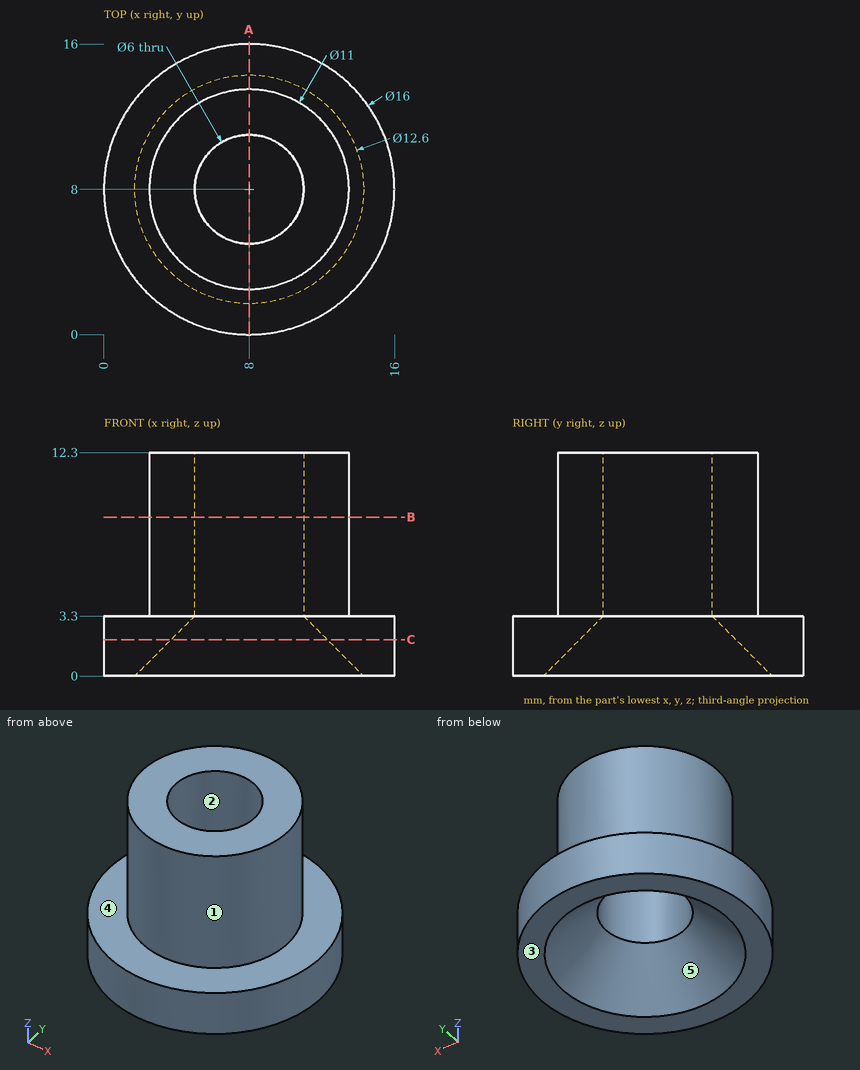
Print and shaded views of the part. All mm, measured from the part's lowest x, y and z. A direction names the side the tool comes from. Round coordinates to 2 decimals unless told otherwise and drop trailing zeros. Write each loop counter-clockwise with the first axis right and the second up, starting at its lowest first coordinate (ties: lowest second). Pieces come first, ordered by that corner, then holes.
(1) Probe line 1 along Y through (x, z) = (8, 7.25); line 2 along Z through (x, y) = (9.5, 15.25); line 3 along Y through (x, z) = (9.75, 4.75). List the from-to ranges inside material, lowest first.
(2) 3-axis set-ups, long thin cutter, end or side, ignore diameter. For the marked faces 4 and 5: which of +Z, -Z, +X, -X, +Y, -Y reach the whole face in a straight line?
(3) Mould opens along X. For the marked faces 1, 2 and 3 say: pulls with the +X half, pulls with the -X half, needs draft (parallel to the pull), parting line crosses it, or undercut.
(4) Slice it at C-C, the plane z = 2. Write the cut outline in (x, y).
(5) Slice it at A-A, the plane x = 8. Write the cut outline in (y, z).
(6) Drop flat-ended pins along their axis: P1, Ø3, axis at x = 10.5, z = 2, coming from the +Y side; P2, Ø2, axis at x = 2, z = 7, coming from the -Y side; P3, Ø2, axis at x = 8, y = 6.5, coming from the +Z side; P4, Ø2, axis at x = 8, z = 10.5, coming from the -Y side. Give the stop position or say it passes through.
(7) Slice it at B-B, the plane z = 8.75. Write the cut outline in (x, y).
From the geometry:
1. line 1: y = 2.5 to 5, 11 to 13.5
1. line 2: z = 0 to 3.3
1. line 3: y = 2.79 to 5.56, 10.44 to 13.21
2. face 4: +Z
2. face 5: -Z
3. face 1: parting line crosses it
3. face 2: undercut
3. face 3: needs draft
4. outline: circle Ø16 at (8, 8); hole circle Ø8.6 at (8, 8)
5. outline: (0, 0) - (1.7, 0) - (5, 3.3) - (5, 12.3) - (2.5, 12.3) - (2.5, 3.3) - (0, 3.3) - close; (11, 3.3) - (14.3, 0) - (16, 0) - (16, 3.3) - (13.5, 3.3) - (13.5, 12.3) - (11, 12.3) - close
6. P1: stops at y = 15.94
6. P2: stops at y = 5.71
6. P3: passes through
6. P4: stops at y = 2.5
7. outline: circle Ø11 at (8, 8); hole circle Ø6 at (8, 8)
